For this review, use the dimensioned drawing (mm, ordinates from the lowest corner) and the shaded views. A direction names the side the tool comes from. Round coordinates to 2 decimals unless told otherwise and drop trailing zeros. Write each loop counter-clockwise with the first axis right and the second up, starting at its lowest first coordinate (ties: lowest second). Pieces come first, ordered by that corner, then holes. Notation, with made-up numbers: M 73.25,71 L 116.25,71 A28 ccw 116.25,110 Z; hole C -28.5,84 d7. An arc over 180 degrees is marked long. One line per question, with ' | ' between items.
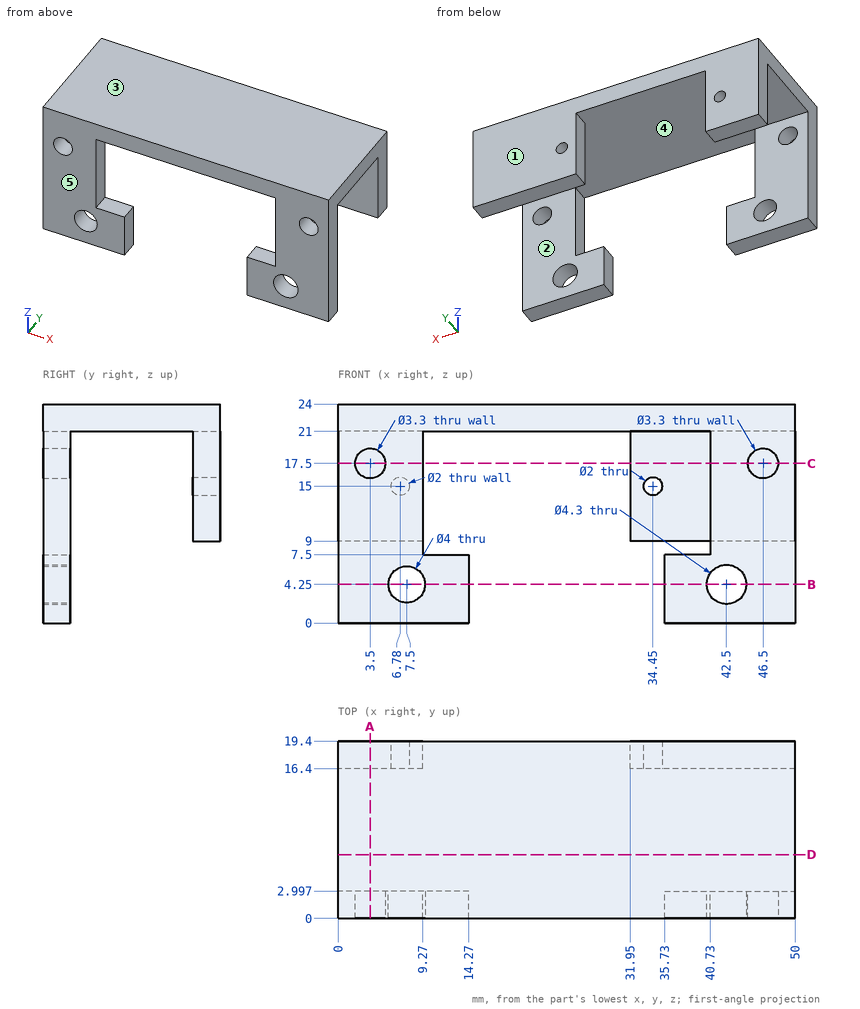
Item 1: Take a section at D-D (y = 7). Write out the cut boundary in (x, z).
Results:
outline: M 0,21 L 50,21 L 50,24 L 0,24 Z
Item 2: To check wall thickness, follow line 1 along X through (y, z) = (0.9, 17.5); line 2 along X through (y, z) = (18.4, 15); line 3 along Z through (x, y) = (7.5, 1). State the ranges of each line that lie inside material, in increasing order. Write a range as from..to.
Results:
line 1: 0..1.85, 5.15..9.27, 40.73..44.85, 48.15..50 | line 2: 0..5.78, 7.78..9.27, 31.95..33.45, 35.45..50 | line 3: 0..2.25, 6.25..24
Item 3: Insertion check: pin 1 Ø2 at (y, z) = (14.5, 7.5) entering from +X; pin 2 Ø0.9 at (x, y) = (37.5, 18.5) entering from -Z; pin 3 Ø1.5 at (x, z) = (35.5, 10.5) entering from -Y; pin 4 Ø1 at (x, z) = (13, 7) entering from +Y. Each pin has a flat end and moves straight along its axis. Give the tip position at first contact, or say it passes through.
Results:
pin 1: through | pin 2: z = 9 | pin 3: y = 16.4 | pin 4: y = 3
Item 4: Take a section at A-A (x = 3.5). Write out the cut boundary in (y, z).
Results:
outline: M 0,0 L 3,0 L 3,15.85 L 0,15.85 Z; M 0,19.15 L 3,19.15 L 3,21 L 16.4,21 L 16.4,9 L 19.4,9 L 19.4,24 L 0,24 Z
Item 5: Mouldability with a two-part tool opening along Y and no side actions: class the marked faces 3, 4 and 5 as +Y half, -Y half, draft (parallel to the pull), parting line (faces both ways), or undercut.
Results:
face 3: draft | face 4: undercut | face 5: -Y half
Item 6: Take a section at B-B (z = 4.25). Write out the cut boundary in (x, y).
Results:
outline: M 0,0 L 5.5,0 L 5.5,3 L 0,3 Z; M 9.5,0 L 14.27,0 L 14.27,3 L 9.5,3 Z; M 35.73,0 L 40.35,0 L 40.35,3 L 35.73,3 Z; M 44.65,0 L 50,0 L 50,3 L 44.65,3 Z
Item 7: Take a section at C-C (z = 17.5). Write out the cut boundary in (x, y), then the cut area to 3 significant figures.
Results:
outline: M 0,0 L 1.85,0 L 1.85,3 L 0,3 Z; M 0,16.4 L 9.27,16.4 L 9.27,19.4 L 0,19.4 Z; M 5.15,0 L 9.27,0 L 9.27,3 L 5.15,3 Z; M 31.95,16.4 L 50,16.4 L 50,19.4 L 31.95,19.4 Z; M 40.73,0 L 44.85,0 L 44.85,3 L 40.73,3 Z; M 48.15,0 L 50,0 L 50,3 L 48.15,3 Z | area: 118 mm2
Item 8: Machinability: for the marked faces 1 and 2, which of the approach directions +Z, -Z, +X, -X, +Y, -Y give a long, thin tool a straight path to every point of the face, cutting with its end or side? Answer none if there is none.
Results:
face 1: +Z, -Z, +X, -X, +Y | face 2: -Z, +X, -X
